```python
from build123d import *

# Parameters (mm, degrees)
SKETCH1_R             = 0.6
BOSS_EXTRUDE1_DEPTH   = 3
BOSS_EXTRUDE1_2_DEPTH = 3
BOSS_EXTRUDE1_3_DEPTH = 3
BOSS_EXTRUDE1_4_DEPTH = 3
BOSS_EXTRUDE2_DEPTH   = 1.3
BOSS_EXTRUDE3_DEPTH   = 3
CIRPATTERN1_COUNT     = 4


# Read off the part's stored shape, not the designer's step: M2 Clearance Hole1
with BuildPart() as part:
    # Sketch1 → Boss-Extrude1 (new body)
    with BuildSketch(Plane(origin=(0, 0, 0), x_dir=(0, 1, 0), z_dir=(0, 0, 1))):
        with BuildLine():
            Line((-1.5, 7.348469228), (-1.5, 37.970383195))
            ThreePointArc((-1.5, 37.970383195), (-26.870057685, 26.870057685), (-37.970383195, 1.5))
            Line((-37.970383195, 1.5), (-7.348469228, 1.5))
            ThreePointArc((-7.348469228, 1.5), (-6.756656365, 3.255394717), (-5.752639047, 4.812187028))
            Line((-5.752639047, 4.812187028), (-7.166852609, 6.226400591))
            Line((-7.166852609, 6.226400591), (-6.226400591, 7.166852609))
            Line((-6.226400591, 7.166852609), (-4.812187028, 5.752639047))
            ThreePointArc((-4.812187028, 5.752639047), (-3.255394717, 6.756656365), (-1.5, 7.348469228))
        make_face()
        with Locations(Location((-12.375, 12.375, 0), (0, 0, 270))):
            Circle(SKETCH1_R, mode=Mode.SUBTRACT)
    extrude(amount=BOSS_EXTRUDE1_DEPTH)

    # Sketch1<9> → Boss-Extrude2 (add)
    with BuildSketch(Plane(origin=(0, 0, 0), x_dir=(0, 1, 0), z_dir=(0, 0, 1))):
        with BuildLine():
            Line((1.5, 7.348469228), (1.5, 37.970383195))
            ThreePointArc((1.5, 37.970383195), (0, 38), (-1.5, 37.970383195))
            Line((-1.5, 37.970383195), (-1.5, 7.348469228))
            ThreePointArc((-1.5, 7.348469228), (0, 7.5), (1.5, 7.348469228))
        make_face()
        with BuildLine():
            ThreePointArc((-37.970383195, 1.5), (-38, 0), (-37.970383195, -1.5))
            Line((-37.970383195, -1.5), (-7.348469228, -1.5))
            ThreePointArc((-7.348469228, -1.5), (-7.5, 0), (-7.348469228, 1.5))
            Line((-7.348469228, 1.5), (-37.970383195, 1.5))
        make_face()
        with BuildLine():
            ThreePointArc((37.970383195, -1.5), (38, 0), (37.970383195, 1.5))
            Line((37.970383195, 1.5), (7.348469228, 1.5))
            ThreePointArc((7.348469228, 1.5), (7.5, 0), (7.348469228, -1.5))
            Line((7.348469228, -1.5), (37.970383195, -1.5))
        make_face()
        with BuildLine():
            ThreePointArc((-1.5, -37.970383195), (0, -38), (1.5, -37.970383195))
            Line((1.5, -37.970383195), (1.5, -7.348469228))
            ThreePointArc((1.5, -7.348469228), (0, -7.5), (-1.5, -7.348469228))
            Line((-1.5, -7.348469228), (-1.5, -37.970383195))
        make_face()
    extrude(amount=BOSS_EXTRUDE2_DEPTH)


with BuildPart() as body_2:
    # Sketch1 → Boss-Extrude1 2 (new body)
    with BuildSketch(Plane(origin=(0, 0, 0), x_dir=(0, 1, 0), z_dir=(0, 0, 1))):
        with BuildLine():
            Line((1.5, 37.970383195), (1.5, 7.348469228))
            ThreePointArc((1.5, 7.348469228), (3.255394717, 6.756656365), (4.812187028, 5.752639047))
            Line((4.812187028, 5.752639047), (6.226400591, 7.166852609))
            Line((6.226400591, 7.166852609), (7.166852609, 6.226400591))
            Line((7.166852609, 6.226400591), (5.752639047, 4.812187028))
            ThreePointArc((5.752639047, 4.812187028), (6.756656365, 3.255394717), (7.348469228, 1.5))
            Line((7.348469228, 1.5), (37.970383195, 1.5))
            ThreePointArc((37.970383195, 1.5), (26.870057685, 26.870057685), (1.5, 37.970383195))
        make_face()
        with Locations(Location((12.375, 12.375, 0), (0, 0, 270))):
            Circle(SKETCH1_R, mode=Mode.SUBTRACT)
    extrude(amount=BOSS_EXTRUDE1_2_DEPTH)

    # M2 Clearance Hole1 4 outline → M2 Clearance Hole1 4 (revolve, cut)
    with BuildSketch(Plane(origin=(-8.485, 8.485, 0), x_dir=(1, 0, 0), z_dir=(0, -1, 0))):
        Polygon((0, 0), (1.2, 0), (1.2, 2.975), (1.225, 3), (0, 3), align=None)
    revolve(axis=Axis((-8.485, 8.485, 0), (0, 0, 1)), mode=Mode.SUBTRACT)



with BuildPart() as body_3:
    # Sketch1 → Boss-Extrude1 3 (new body)
    with BuildSketch(Plane(origin=(0, 0, 0), x_dir=(0, 1, 0), z_dir=(0, 0, 1))):
        with BuildLine():
            Line((-7.348469228, -1.5), (-37.970383195, -1.5))
            ThreePointArc((-37.970383195, -1.5), (-26.870057685, -26.870057685), (-1.5, -37.970383195))
            Line((-1.5, -37.970383195), (-1.5, -7.348469228))
            ThreePointArc((-1.5, -7.348469228), (-3.255394717, -6.756656365), (-4.812187028, -5.752639047))
            Line((-4.812187028, -5.752639047), (-6.226400591, -7.166852609))
            Line((-6.226400591, -7.166852609), (-7.166852609, -6.226400591))
            Line((-7.166852609, -6.226400591), (-5.752639047, -4.812187028))
            ThreePointArc((-5.752639047, -4.812187028), (-6.756656365, -3.255394717), (-7.348469228, -1.5))
        make_face()
        with Locations(Location((-12.375, -12.375, 0), (0, 0, 270))):
            Circle(SKETCH1_R, mode=Mode.SUBTRACT)
    extrude(amount=BOSS_EXTRUDE1_3_DEPTH)

    # M2 Clearance Hole1 2 outline → M2 Clearance Hole1 2 (revolve, cut)
    with BuildSketch(Plane(origin=(8.485, -8.485, 0), x_dir=(1, 0, 0), z_dir=(0, -1, 0))):
        Polygon((0, 0), (1.2, 0), (1.2, 2.975), (1.225, 3), (0, 3), align=None)
    revolve(axis=Axis((8.485, -8.485, 0), (0, 0, 1)), mode=Mode.SUBTRACT)


with BuildPart() as body_4:
    # Sketch1 → Boss-Extrude1 4 (new body)
    with BuildSketch(Plane(origin=(0, 0, 0), x_dir=(0, 1, 0), z_dir=(0, 0, 1))):
        with BuildLine():
            Line((37.970383195, -1.5), (7.348469228, -1.5))
            ThreePointArc((7.348469228, -1.5), (6.756656365, -3.255394717), (5.752639047, -4.812187028))
            Line((5.752639047, -4.812187028), (7.166852609, -6.226400591))
            Line((7.166852609, -6.226400591), (6.226400591, -7.166852609))
            Line((6.226400591, -7.166852609), (4.812187028, -5.752639047))
            ThreePointArc((4.812187028, -5.752639047), (3.255394717, -6.756656365), (1.5, -7.348469228))
            Line((1.5, -7.348469228), (1.5, -37.970383195))
            ThreePointArc((1.5, -37.970383195), (26.870057685, -26.870057685), (37.970383195, -1.5))
        make_face()
        with Locations(Location((12.375, -12.375, 0), (0, 0, 270))):
            Circle(SKETCH1_R, mode=Mode.SUBTRACT)
    extrude(amount=BOSS_EXTRUDE1_4_DEPTH)

    # M2 Clearance Hole1 outline → M2 Clearance Hole1 (revolve, cut)
    with BuildSketch(Plane(origin=(8.485, 8.485, 0), x_dir=(1, 0, 0), z_dir=(0, -1, 0))):
        Polygon((0, 0), (1.2, 0), (1.2, 2.975), (1.225, 3), (0, 3), align=None)
    revolve(axis=Axis((8.485, 8.485, 0), (0, 0, 1)), mode=Mode.SUBTRACT)


with BuildPart() as boss_extrude2_piece_1:
    # of the separate pieces the step leaves, piece 1, a body of its own (boss_extrude2_pieces)
    add(part.part.solids().sort_by_distance((-37.970383195, -1.5, 1.3))[0])

    # M2 Clearance Hole1 3 outline → M2 Clearance Hole1 3 (revolve, cut)
    with BuildSketch(Plane(origin=(-8.485, -8.485, 0), x_dir=(1, 0, 0), z_dir=(0, -1, 0))):
        Polygon((0, 0), (1.2, 0), (1.2, 2.975), (1.225, 3), (0, 3), align=None)
    revolve(axis=Axis((-8.485, -8.485, 0), (0, 0, 1)), mode=Mode.SUBTRACT)


with BuildPart() as boss_extrude2_piece_2:
    # of the separate pieces the step leaves, piece 2, a body of its own (boss_extrude2_pieces)
    add(part.part.solids().sort_by_distance((-1.5, 7.348469228, 0))[0])


with BuildPart() as boss_extrude2_piece_3:
    # of the separate pieces the step leaves, piece 3, a body of its own (boss_extrude2_pieces)
    add(part.part.solids().sort_by_distance((37.970383195, -1.5, 0))[0])


with BuildPart() as body_2_1:
    add(body_2.part)

    add(body_3.part)  # Boss-Extrude3 merges body 3

    add(body_4.part)  # Boss-Extrude3 merges body 4

    add(boss_extrude2_piece_1.part)  # Boss-Extrude3 merges Boss-Extrude2 piece 1

    add(boss_extrude2_piece_2.part)  # Boss-Extrude3 merges Boss-Extrude2 piece 2

    add(boss_extrude2_piece_3.part)  # Boss-Extrude3 merges Boss-Extrude2 piece 3
    # Sketch1<10> → Boss-Extrude3 (add)
    with BuildSketch(Plane(origin=(0, 0, 0), x_dir=(0, 1, 0), z_dir=(0, 0, 1))):
        with BuildLine():
            Line((-1.5, -7.348469228), (-1.5, -8.7))
            Line((-1.5, -8.7), (1.5, -8.7))
            Line((1.5, -8.7), (1.5, -7.348469228))
            ThreePointArc((1.5, -7.348469228), (0, -7.5), (-1.5, -7.348469228))
        make_face()
        with BuildLine():
            Line((-7.348469228, 1.5), (-8.7, 1.5))
            Line((-8.7, 1.5), (-8.7, -1.5))
            Line((-8.7, -1.5), (-7.348469228, -1.5))
            ThreePointArc((-7.348469228, -1.5), (-7.5, 0), (-7.348469228, 1.5))
        make_face()
        with BuildLine():
            Line((1.5, 8.7), (-1.5, 8.7))
            Line((-1.5, 8.7), (-1.5, 7.348469228))
            ThreePointArc((-1.5, 7.348469228), (0, 7.5), (1.5, 7.348469228))
            Line((1.5, 7.348469228), (1.5, 8.7))
        make_face()
        with BuildLine():
            Line((8.7, -1.5), (8.7, 1.5))
            Line((8.7, 1.5), (7.348469228, 1.5))
            ThreePointArc((7.348469228, 1.5), (7.5, 0), (7.348469228, -1.5))
            Line((7.348469228, -1.5), (8.7, -1.5))
        make_face()
    extrude(amount=BOSS_EXTRUDE3_DEPTH)

    # Sketch8 → CBORE for M2 SHCS1 (revolve, cut)
    with BuildSketch(Plane(origin=(25.809397513, 25.809397513, 3), x_dir=(0, -1, 0), z_dir=(1, 0, 0))):
        Polygon((0, 0), (0, 3), (1.2, 3), (1.2, 2), (2.2, 2), (2.2, 0.025), (2.225, 0), align=None)
    cbore_for_m2_shcs1 = revolve(axis=Axis((25.809397513, 25.809397513, 9.35), (0, 0, -1)), mode=Mode.SUBTRACT)

    # CirPattern1: CBORE for M2 SHCS1 ×4 about axis
    cirpattern1_axis = Axis((0, 0, 0), (0, 0, 1))
    for i in range(1, CIRPATTERN1_COUNT):
        add(cbore_for_m2_shcs1.rotate(cirpattern1_axis, i * 360 / CIRPATTERN1_COUNT), mode=Mode.SUBTRACT)


solid = body_2_1.part
```
Could you check a few things on this model? Use its own coordinates, in mm. A direction names the side the tool comes from. Round coordinates to 2 decimals unless told otherwise and drop trailing zeros. Write each loop counter-clockwise with the first axis right and the second up, starting at its lowest first coordinate (ties: lowest second). Pieces come first, ordered by that corner, then holes.
(1) For pin 1 (0.8 mm diameter, centred on y = 23.5, z = 2.5, fed in from -X); pin 2 (1.1 mm diameter, centred on x = 12.375, y = 12.375, fed in from +Z); pin 3 (3.5 mm diameter, centred on x = -26, y = 26, fed in from +Z); pin 4 (1 mm diameter, centred on x = -4, z = 2, fed in from +Y), each with a flat end and sliding along its axis, tell me the tip position at first contact or that it passes through.
Findings below:
pin 1: stops at x = -30.17
pin 2: passes through
pin 3: stops at z = 1
pin 4: stops at y = 37.84
(2) Suppose I cut it at D-D on z = 2.5. State how many separate pieces and enclosed holes the cut face has, and give its area (3 significant figures).
Findings below:
separate pieces: 1
enclosed holes: 9
area: 3,920 mm2
(3) Thinking about a two-plate mould opening in Y: for faces 1 (the face through (8.7, 0, 2)), 2 (the face through (1.5, -23, 2)), 3 (the face through (0.1, -7.5, 1.5)), which applies, +Y half, -Y half, draft (parallel to the pull), parting line (faces both ways), or undercut?
Findings below:
face 1: undercut
face 2: draft
face 3: undercut
(4) Suppose I cut it at B-B on x = 17. Write out the boundary of the cut face in (y, z).
Findings below:
outline: (-33.99, 0) - (33.99, 0) - (33.99, 3) - (1.5, 3) - (1.5, 1.3) - (-1.5, 1.3) - (-1.5, 3) - (-33.99, 3) - close
(5) Suppose I cut it at C-C on y = -30.5. Write out the boundary of the cut face in (x, z), and give its area (3 significant figures).
Findings below:
outline: (-22.67, 0) - (22.67, 0) - (22.67, 3) - (1.5, 3) - (1.5, 1.3) - (-1.5, 1.3) - (-1.5, 3) - (-22.67, 3) - close
area: 131 mm2
(6) If I drill on probe 1 along X at (y, z) = (8, 0.55); probe 2 along X at (y, z) = (25.5, 1.4); probe 3 along X at (y, z) = (-24, 2.3), over which ranges is the centre line in solid material (lowest first)?
Findings below:
probe 1: x = -37.15 to -9.58, -7.39 to 7.39, 9.58 to 37.15
probe 2: x = -28.17 to -27.99, -23.63 to -1.5, 1.5 to 23.63, 27.99 to 28.17
probe 3: x = -29.46 to -27.06, -24.56 to -1.5, 1.5 to 24.56, 27.06 to 29.46
(7) Suppose I cut it at A-A on y = 0. Write out the boundary of the cut face in (x, z).
Findings below:
outline: (-38, 0) - (-7.5, 0) - (-7.5, 3) - (-8.7, 3) - (-8.7, 1.3) - (-38, 1.3) - close; (7.5, 0) - (38, 0) - (38, 1.3) - (8.7, 1.3) - (8.7, 3) - (7.5, 3) - close
(8) Which directions (+Z, -Z, +X, -X, +Y, -Y) give clear straight access to the entire face, cutting with the end or side of a thin tool? Please do faces 4 (the face through (1.5, 24, 2)), 5 (the face through (-23, -1.5, 2)), 6 (the face through (0, -24, 1.3)), 7 (the face through (24.8, -24.8, 1)).
Findings below:
face 4: +Z, +Y
face 5: +Z, -X
face 6: +Z, -Y
face 7: +Z
